Source: CAD feature listing. Evaluate the final solid. Frame: model axes, mm. Face numbers are marked on the shaded views. Round coordinates to 2 decimals unless told otherwise and drop trailing zeros. Write each loop counter-clockwise with the first axis right and the second up, starting at its lowest first coordinate (ties: lowest second). Pieces come first, ordered by that corner, then holes. Notation, with made-up numbers: M 24,-22 L 29,-22 A20 ccw 29,12 Z; hole C 23.5,-5 d11. An arc over 180 degrees is marked long. Answer in a Markdown table with one row per item. Add a question column.
Item 1: Mould query, pull axis Y, two halves, no side actions, for the marked faces 1, 2 and 3. Classes: released by +Y, released by -Y, zero draft, split by the parting line, or undercut.
Item 2: Cut plane C-C on z = 57. Return loops of the section in (x, y).
Item 3: Cut plane A-A on y = -60. Give the number of separate pieces and of enclosed holes in the cut face, and give its area (3 significant figures).
Item 4: Contact query for flat-ended pins moving along their axis: pin 1 (9.5 mm diameter, centred on y = 0, z = 128, fed in from -X); pin 2 (12 mm diameter, centred on y = 11.5, z = 252, fed in from +X); pin 3 (10 mm diameter, centred on x = 74, y = -38.5, fed in from +Z); pin 4 (3 mm diameter, centred on y = -55.5, z = 221.5, fed in from -X). Output: stop coordinate, or through.
Item 5: Cut plane B-B on x = 260. Return loops of the section in (y, z), and give its area (3 significant figures).
Item 6: Cut plane D-D on x = 161.5. Return loops of the section in (y, z), and give its area (3 significant figures).
Item 7: Material intervals for probe 1 along Y at (x, z) = (260, 5); probe 2 along Z at (x, y) = (217.5, 75), sorted ascending.
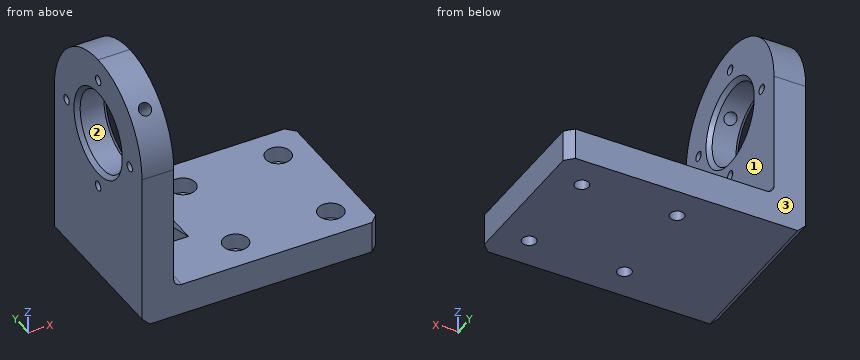
from build123d import *

# Parameters (mm, degrees)
F1_DEPTH        = 100
F2_R            = 99.99999
F3_SIZE         = 10
F5_DEPTH        = 25
F6_R            = 50
F7_DEPTH        = 40.001
F10_D           = 12.1
F11_D           = 15.5
F11_DEPTH       = 70
F11_START       = 0.3007608
F11_TIP         = 4.6566697975
F13_D           = 17.5
F13_CBORE_D     = 31.5
F13_CBORE_DEPTH = 20
F14_SIZE        = 5
F15_R           = 10


# Not quite as in the source:
# - a fillet or chamfer is up to 0.001 mm smaller than in the source, because OpenCascade refuses the exact size


with BuildPart() as f1:
    # F0 (on Front) → F1 (new body, symmetric)
    with BuildSketch(Plane.XZ):
        Polygon((40, 300), (0, 300), (0, 0), (300, 0), (300, 40), (40, 40), align=None)
    extrude(amount=F1_DEPTH, both=True)

    # F2 (radius 100 in the source; OpenCascade refuses exactly that, so slightly less here)
    f2_edges = [f1.edges().sort_by_distance(p)[0] for p in [
        (20, -100, 300),
        (20, 100, 300),
    ]]
    fillet(f2_edges, radius=F2_R)

    # F3
    f3_edges = [f1.edges().sort_by_distance(p)[0] for p in [
        (300, -100, 20),
        (300, 100, 20),
        (0, 0, 0),
    ]]
    chamfer(f3_edges, length=F3_SIZE)

    # F4 (on Front) → F5 (join, symmetric)
    with BuildSketch(Plane.XZ):
        Polygon((40, 100), (40, 40), (100, 40), align=None)
    extrude(amount=F5_DEPTH, both=True)

    # F6 (on face) → F7 (cut, through all)
    with BuildSketch(Plane.YZ.offset(40)):
        with Locations((0, 200)):
            Circle(F6_R)
    extrude(amount=-F7_DEPTH, mode=Mode.SUBTRACT)

    # F10 (through all)
    with Locations(Plane.YZ.offset(40)):
        with Locations((0, 272), (72, 200), (0, 128), (-72, 200)):
            Hole(F10_D / 2)

    # F11
    # its depths count from where the whole tool has entered the part; down to there all is cleared
    with Locations(Plane(origin=(0, -170.7106781187, 170.7106781187), x_dir=(1, 0, 0), z_dir=(0, -0.7071067812, 0.7071067812)).offset(-F11_START)):
        with Locations((20, 141.4213562373)):
            Hole(F11_D / 2, depth=F11_DEPTH)
            with Locations((0, 0, -(F11_DEPTH + F11_TIP / 2))):  # 118° drill point
                Cone(0, F11_D / 2, F11_TIP, mode=Mode.SUBTRACT)

    # F13 (through all)
    with Locations(Plane.XY.offset(40)):
        with Locations((140, -60), (140, 60), (260, 60), (260, -60)):
            CounterBoreHole(F13_D / 2, F13_CBORE_D / 2, F13_CBORE_DEPTH)

    # F14
    f14_edges = [f1.edges().sort_by_distance(p)[0] for p in [
        (40, -50, 200),
        (0, -50, 200),
    ]]
    chamfer(f14_edges, length=F14_SIZE)

    # F15
    f15_edges = [f1.edges().sort_by_distance(p)[0] for p in [
        (40, -62.5, 40),
        (40, 62.5, 40),
    ]]
    fillet(f15_edges, radius=F15_R)


solid = f1.part
Results below:
| question | item | result |
|---|---|---|
| 1 | face 1 | zero draft |
| 1 | face 2 | undercut |
| 1 | face 3 | released by +Y |
| 2 | outline | M 0,-100 L 40,-100 L 40,-25 L 83,-25 L 83,25 L 40,25 L 40,100 L 0,100 Z |
| 3 | separate pieces | 3 |
| 3 | enclosed holes | 1 |
| 3 | area | 19,300 mm2 |
| 4 | pin 1 | through |
| 4 | pin 2 | x = 40 |
| 4 | pin 3 | z = 40 |
| 4 | pin 4 | x = 0 |
| 5 | outline | M -100,0 L -68.75,0 L -68.75,20 L -75.75,20 L -75.75,40 L -100,40 Z; M -51.25,0 L 51.25,0 L 51.25,20 L 44.25,20 L 44.25,40 L -44.25,40 L -44.25,20 L -51.25,20 Z; M 68.75,0 L 100,0 L 100,40 L 75.75,40 L 75.75,20 L 68.75,20 Z |
| 5 | area | 6,040 mm2 |
| 6 | outline | M -100,0 L 100,0 L 100,40 L -100,40 Z |
| 6 | area | 8,000 mm2 |
| 7 | probe 1 | -100 to -68.75, -51.25 to 51.25, 68.75 to 100 |
| 7 | probe 2 | 0 to 40 |
